from build123d import *

# Parameters (mm, degrees)
F1_W     = 20
F1_H     = 3
F2_DEPTH = 3


with BuildPart() as f2:
    # F1 (on Front) → F2 (new body)
    with BuildSketch(Plane.XZ):
        Polygon((-60, -20), (60, -20), (60, -3), (50, -3), (50, 0), (60, 0), (60, 17), (50, 17), (50, 20), (40, 20), (40, 17), (20, 17), (20, 20), (10, 20), (10, 17), (-10, 17), (-10, 20), (-20, 20), (-20, 17), (-40, 17), (-40, 20), (-50, 20), (-50, 17), (-60, 17), (-60, 0), (-50, 0), (-50, -3), (-60, -3), align=None)
        with Locations((-30, -1.5)):
            Rectangle(F1_W, F1_H, mode=Mode.SUBTRACT)
        with Locations((0, -1.5)):
            Rectangle(F1_W, F1_H, mode=Mode.SUBTRACT)
        with Locations((30, -1.5)):
            Rectangle(F1_W, F1_H, mode=Mode.SUBTRACT)
    extrude(amount=-F2_DEPTH)


solid = f2.part
Input: part model. Units: mm. Frame: model coordinates. A direction names the side the tool comes from. Round coordinates to 2 decimals unless told otherwise and drop trailing zeros. Write each loop counter-clockwise with the first axis right and the second up, starting at its lowest first coordinate (ties: lowest second). Pieces come first, ordered by that corner, then holes.
1) Contact query for flat-ended pins moving along their axis: P1, Ø1.5, axis at x = 31, y = 1.5, coming from the +Z side; P2, Ø0.9, axis at y = 2, z = 18.5, coming from the -X side; P3, Ø0.9, axis at y = 2, z = -2, coming from the +X side. Output: stop coordinate, or through.
2) Reachability of faces 1 (the flat face through (30, 1, 17)), 2 (the flat face through (10, 1, -2)), 3 (the flat face through (55, 1, 17)), 4 (the flat face through (-55, 1, 0)) from +Z, -Z, +X, -X, +Y, -Y: full face, straight path, thin tool, end or side. Return the list, or none.
3) Cut plane B-B (y = 2.55). Count the separate pieces of the cut face and the enclosed holes in it, then the cut area to 3 significant figures.
4) Ray query, L1, parallel to X at y = 0.6, z = 18; L2, parallel to Z at x = -30.5, y = 2.5. Return the intervals inside material, ascending.
5) Draft query along Z for faces 5 (the flat face through (-20, 1, -2)), 6 (the flat face through (-30, 1, 17)), 7 (the flat face through (20, 1, 18)). Return one class per face: pulls with the +Z half, pulls with the -Z half, needs draft (parallel to the pull), parting line crosses it, or undercut.
6) Cut plane A-A (x = -33). Return the cut outline in (y, z).
Geometry says:
1. P1: stops at z = 17
1. P2: stops at x = -50
1. P3: stops at x = 50
2. face 1: +Z, +Y, -Y
2. face 2: +Y, -Y
2. face 3: +Z, +X, +Y, -Y
2. face 4: -X, +Y, -Y
3. separate pieces: 1
3. enclosed holes: 3
3. area: 4,320 mm2
4. L1: x = -50 to -40, -20 to -10, 10 to 20, 40 to 50
4. L2: z = -20 to -3, 0 to 17
5. face 5: undercut
5. face 6: pulls with the +Z half
5. face 7: needs draft
6. outline: (0, -20) - (3, -20) - (3, -3) - (0, -3) - close; (0, 0) - (3, 0) - (3, 17) - (0, 17) - close
